```python
from build123d import *

# Parameters (mm, degrees)
F2_R = 6.34999
F3_R = 5.08


# Not quite as in the source:
# - a fillet or chamfer is up to 0.001 mm smaller than in the source, because OpenCascade refuses the exact size


with BuildPart() as f1:
    # F0 (on Front) → F1 (revolve)
    with BuildSketch(Plane.XZ):
        Polygon((-63.5, 0), (0, 0), (0, 12.7), (-50.8, 12.7), (-50.8, 127), (-63.5, 127), align=None)
    revolve(axis=Axis((0, 0, 6.35), (0, 0, -1)))

    # F2 (radius 6.35 in the source; OpenCascade refuses exactly that, so slightly less here)
    f2_edges = [f1.edges().sort_by_distance(p)[0] for p in [
        (63.5, 0, 127),
        (50.8, 0, 127),
    ]]
    fillet(f2_edges, radius=F2_R)

    # F3
    f3_edges = [f1.edges().sort_by_distance(p)[0] for p in [
        (63.5, 0, 0),
    ]]
    fillet(f3_edges, radius=F3_R)


solid = f1.part
```
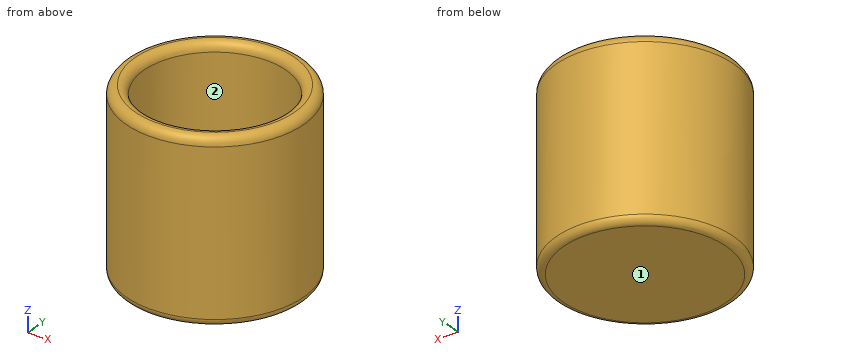
Part model, mm, in its own coordinate system. Face numbers are marked on the shaded views. A direction names the side the tool comes from. Give positions to 0.01 mm unless a question says otherwise; leave off trailing zeros. Order: outer loops, then holes, each group sorted by start corner. A loop starts at its lowest first (then second) coordinate and runs counter-clockwise, first axis right, second up. Notation, with made-up numbers: M 17.25,40 L 21.25,40 A18 ccw 21.25,46 Z; hole C 0,-5 d6. An arc over 180 degrees is marked long. Use a Markdown table: item, result. Add a question column.
(1) 3-axis set-ups, long thin cutter, end or side, ignore diameter. For the marked faces 1 and 2: which of +Z, -Z, +X, -X, +Y, -Y reach the whole face in a straight line?
(2) Saw through at C-C, the plane z = 99.5. Give the cut face in (x, y).
(3) Drop flat-ended pins along their axis: P1, Ø4, axis at x = 46.5, y = 8.5, coming from the +Z side; P2, Ø8, axis at y = -12.5, z = 104.5, coming from the -X side; P3, Ø1.5, axis at y = -45, z = 16, coming from the -X side. Give the stop position or say it passes through.
(4) Probe line 1 along Y through (x, z) = (0, 79.5); line 2 along Y through (x, z) = (20, 81.5); line 3 along Z through (x, y) = (-3, -2.5). List the from-to ranges inside material, lowest first. Write a range as [from, to].
Answer key:
| question | item | result |
|---|---|---|
| 1 | face 1 | -Z, +X, -X, +Y, -Y |
| 1 | face 2 | +Z |
| 2 | outline | C 0,0 d127; hole C 0,0 d101.6 |
| 3 | P1 | z = 12.7 |
| 3 | P2 | x = -62.93 |
| 3 | P3 | x = -45.54 |
| 4 | line 1 | [-63.5, -50.8], [50.8, 63.5] |
| 4 | line 2 | [-60.27, -46.7], [46.7, 60.27] |
| 4 | line 3 | [0, 12.7] |
